Can you work these out from the model? Positions are in its coordinate system, mm. A direction names the side the tool comes from. Coordinates: 2 decimals unless noted, no trailing zeros. Loops run counter-clockwise (first coordinate to the right, second up) from the corner with the lowest first, then second, coordinate; pieces in that order, holes last. Notation, with made-up numbers: (-39, 0) -> (-20, 0) arc R9 cw to (-20, 5) -> close; hole circle Ø9 at (17.5, -40). An arc over 180 degrees is marked (long way). Put each result on its own line as item: value. Start each with the question number.
Item 1: If we section it at B-B on z = 0: Please give me the cut outline in (x, y).
Item 2: We'd pull the mould along X, two halves only. Please class faces 1 (the flat face through (13, 28, -5)), 2 (the cylindrical face through (-36.39, 3.94, -0.98)), 3 (the flat face through (-24.49, 3.94, -17)), 4 (the flat face through (24.49, 3.94, 17)): pulls with the +X half, pulls with the -X half, needs draft (parallel to the pull), parting line crosses it, or undercut.
Item 3: For faces 5 (the cylindrical face through (-10.74, 12.81, -2.38)), 6 (the cylindrical face through (-15.62, 26.48, -3.47)), which set-ups out of +Z, -Z, +X, -X, +Y, -Y let a thin tool reach every point of the face, with its end or its side?
Item 4: If we section it at C-C on x = -32: Please give me the cut outline in (y, z), plus the area to 3 significant figures.
Item 5: If we section it at D-D on z = -17: Please give me the cut outline in (x, y), plus the area to 3 significant figures.
Item 6: Please list where these lines run through material, in increasing order: L1, parallel to X at y = 2.5, z = 0; L2, parallel to X at y = 10.25, z = 0; L3, parallel to Y at x = -7.5, z = -18. Write a range as from..to.
Item 7: Will these pins go through, and if not, where does the flat tip stop? P1, Ø11, axis at x = 3, z = -3.5, coming from the +Y side; P2, Ø2, axis at y = 3, z = -12, coming from the -X side; P3, Ø1.5, axis at y = 9, z = 14, coming from the +X side; P4, Ø15.5, axis at x = 12.5, z = 11, coming from the +Y side.
Item 8: If we section it at A-A on x = 0: Please give me the cut outline in (y, z), plus the area to 3 significant figures.
```python
from build123d import *

# Parameters (mm, degrees)
SKETCH_1_R      = 4.5
SKETCH_1_R_2    = 11
EXTRUDE_1_DEPTH = 8
CHAMFER_1_SIZE  = 1.5


with BuildPart() as part:
    # 草图1 → 凸台-拉伸1 (new body)
    with BuildSketch(Plane(origin=(0, 0, 0), x_dir=(1, 0, 0), z_dir=(0, 1, 0))):
        with BuildLine():
            Line((-37.25, 10.790620927), (-11.375, 23.379678676))
            ThreePointArc((-11.375, 23.379678676), (0, 26), (11.375, 23.379678676))
            Line((11.375, 23.379678676), (37.25, 10.790620927))
            ThreePointArc((37.25, 10.790620927), (44, 0), (37.25, -10.790620927))
            Line((37.25, -10.790620927), (11.375, -23.379678676))
            ThreePointArc((11.375, -23.379678676), (0, -26), (-11.375, -23.379678676))
            Line((-11.375, -23.379678676), (-37.25, -10.790620927))
            ThreePointArc((-37.25, -10.790620927), (-44, 0), (-37.25, 10.790620927))
        make_face()
        with Locations(Location((-32, 0, 0), (0, 0, 270))):
            Circle(SKETCH_1_R, mode=Mode.SUBTRACT)
        with Locations(Location((32, 0, 0), (0, 0, 270))):
            Circle(SKETCH_1_R, mode=Mode.SUBTRACT)
        with Locations(Location((0, 0, 0), (0, 0, 270))):
            Circle(SKETCH_1_R_2, mode=Mode.SUBTRACT)
    extrude(amount=EXTRUDE_1_DEPTH)

    # 草图2 → 旋转1 (revolve)
    with BuildSketch(Plane(origin=(0, 0, 0), x_dir=(0, 0, -1), z_dir=(1, 0, 0))):
        with BuildLine():
            Line((-18, 8), (-11, 8))
            Line((-11, 8), (-11, 23.801960973))
            ThreePointArc((-11, 23.801960973), (-12.550632728, 25.7852804), (-13.747727085, 28))
            Line((-13.747727085, 28), (-16, 28))
            Line((-16, 28), (-16, 25))
            Line((-16, 25), (-18, 25))
            Line((-18, 25), (-18, 8))
        make_face()
    revolve(axis=Axis((0, 0, 0), (0, 1, 0)))

    # 倒角1
    chamfer_1_edges = [part.edges().sort_by_distance(p)[0] for p in [
        (0, 0, -11),
    ]]
    chamfer(chamfer_1_edges, length=CHAMFER_1_SIZE)


solid = part.part
```
Solutions:
1. outline: (-44, 0) -> (-36.5, 0) -> (-36.5, 8) -> (-44, 8) -> close; (-27.5, 0) -> (-12.5, 0) -> (-11, 1.5) -> (-11, 23.8) arc R15 cw to (-13.75, 28) -> (-16, 28) -> (-16, 25) -> (-18, 25) -> (-18, 8) -> (-27.5, 8) -> close; (11, 1.5) -> (12.5, 0) -> (27.5, 0) -> (27.5, 8) -> (18, 8) -> (18, 25) -> (16, 25) -> (16, 28) -> (13.75, 28) arc R15 cw to (11, 23.8) -> close; (36.5, 0) -> (44, 0) -> (44, 8) -> (36.5, 8) -> close
2. face 1: needs draft
2. face 2: undercut
2. face 3: pulls with the -X half
2. face 4: pulls with the +X half
3. face 5: +Y, -Y
3. face 6: +Y
4. outline: (0, -13.34) -> (8, -13.34) -> (8, -4.5) -> (0, -4.5) -> close; (0, 4.5) -> (8, 4.5) -> (8, 13.34) -> (0, 13.34) -> close
4. area: 142 mm^2
5. outline: (-24.49, 0) -> (24.49, 0) -> (24.49, 8) -> (5.92, 8) -> (5.92, 25) -> (-5.92, 25) -> (-5.92, 8) -> (-24.49, 8) -> close
5. area: 593 mm^2
6. L1: -44..-36.5, -27.5..-11, 11..27.5, 36.5..44
6. L2: -18..-11, 11..18
6. L3: 0..8
7. P1: through
7. P2: x = -36.82
7. P3: x = 12.18
7. P4: y = 28
8. outline: (0, -26) -> (8, -26) -> (8, -18) -> (25, -18) -> (25, -16) -> (28, -16) -> (28, -13.75) arc R15 cw to (23.8, -11) -> (1.5, -11) -> (0, -12.5) -> close; (0, 12.5) -> (1.5, 11) -> (23.8, 11) arc R15 cw to (28, 13.75) -> (28, 16) -> (25, 16) -> (25, 18) -> (8, 18) -> (8, 26) -> (0, 26) -> close
8. area: 493 mm^2
